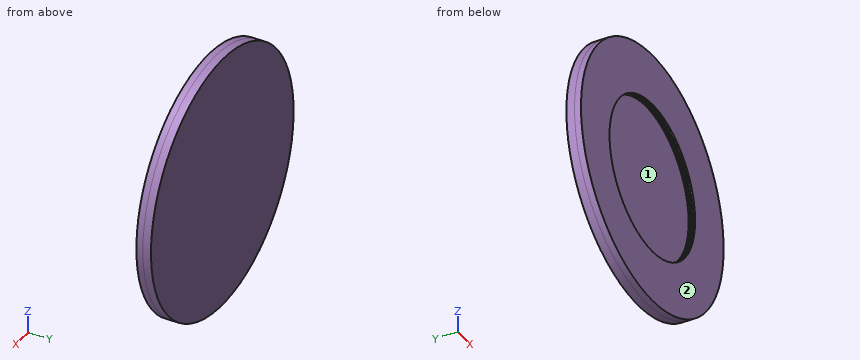
```python
from build123d import *

# Parameters (mm, degrees)
SKETCH1_R           = 15.875
BOSS_EXTRUDE1_DEPTH = 1
BOSS_EXTRUDE2_START = 0.8
SKETCH2_R           = 15.875
SKETCH2_R_2         = 9.525
BOSS_EXTRUDE2_DEPTH = 0.8
THREAD1_PITCH       = 0.25


with BuildPart() as part:
    # Sketch1 → Boss-Extrude1 (new body)
    with BuildSketch(Plane(origin=(0, 0, 0), x_dir=(1, 0, 0), z_dir=(0, 1, 0))):
        with Locations(Location((0, 0, 0), (0, 0, 270))):
            Circle(SKETCH1_R)
    extrude(amount=BOSS_EXTRUDE1_DEPTH)

    # Sketch2 → Boss-Extrude2 (add)
    with BuildSketch(Plane.XZ.offset(BOSS_EXTRUDE2_START)):
        with Locations(Location((0, 0, 0), (0, 0, 270))):
            Circle(SKETCH2_R)
        with Locations(Location((0, 0, 0), (0, 0, 270))):
            Circle(SKETCH2_R_2, mode=Mode.SUBTRACT)
    extrude(amount=-BOSS_EXTRUDE2_DEPTH)

    # Thread1: the profile of Thread Profile1 profile screwed along a right-hand helix of 4 turns, 6 arcs to a turn; built about Z, then put on its axis
    thread1_z = Axis((0, 0, 0), (0, 0, 1))
    thread1_corners = [(9.5247, 0, -0.000173205), (9.660316469, 0, 0.078125), (9.660316469, 0, 0.109375), (9.5247, 0, 0.187673204)]
    with BuildLine(mode=Mode.PRIVATE) as thread1_profile:
        Line(thread1_corners[0], thread1_corners[1])
        Line(thread1_corners[1], thread1_corners[2])
        Line(thread1_corners[2], thread1_corners[3])
        Line(thread1_corners[3], thread1_corners[0])
    thread1_cap = Face(thread1_profile.wire())
    thread1_turn_angles = [0, 30, 60, 90, 120, 150, 180, 210, 240, 270, 300, 330, 360]
    thread1_turn_weights = [1, 0.8660254037844387, 1, 0.8660254037844387, 1, 0.8660254037844387, 1, 0.8660254037844387, 1, 0.8660254037844387, 1, 0.8660254037844387, 1]
    thread1_turn_rails = [Edge.make_bspline([Vector(p[0], p[1], 0).rotate(thread1_z, thread1_turn_angles[k]) / thread1_turn_weights[k] + Vector(0, 0, p[2] + THREAD1_PITCH * thread1_turn_angles[k] / 360) for k in range(13)], [0, 0, 0, 1, 1, 2, 2, 3, 3, 4, 4, 5, 5, 6, 6, 6], 2, thread1_turn_weights) for p in thread1_corners]
    thread1_turn_sides = [Face.make_surface_from_curves(thread1_turn_rails[p[0]], thread1_turn_rails[p[1]]) for p in [(0, 1), (1, 2), (2, 3), (3, 0)]]
    thread1 = Plane(origin=(0, -0.8, 0), x_dir=(1, 0, 0), z_dir=(0, 1, 0)) * Solid(Shell([*[p.moved(Location((0, 0, THREAD1_PITCH * i))) for i in range(4) for p in thread1_turn_sides], thread1_cap, thread1_cap.rotate(thread1_z, 1440).moved(Location((0, 0, THREAD1_PITCH * 1440 / 360)))]))
    add(thread1, mode=Mode.SUBTRACT)


solid = part.part
```
Check sheet for the modelled part. Datum: model origin and axes. Units: mm. Face numbers are marked on the shaded views. Give positions to 0.01 mm unless a question says otherwise; leave off trailing zeros. Order: outer loops, then holes, each group sorted by start corner. A loop starts at its lowest first (then second) coordinate and runs counter-clockwise, first axis right, second up. Notation, with made-up numbers: (84.5, 65.5) -> (143.5, 65.5) arc R21 cw to (143.5, 94.5) -> close; hole circle Ø3 at (68, -24). An arc over 180 degrees is marked (long way). Use CSV: the item, a comma, the result in double quotes. Start each with the question number.
1) Mould release check, pull along X, two halves, no side actions. Record for the marked faces 1 and 2: released by +X, released by -X, zero draft, split by the parting line, or undercut.
2) Material ranges on line 1 (Y direction, x = -4.5, z = -2.5); line 2 (X direction, y = -0.25, z = 4); line 3 (Z direction, x = 0, y = -0.7) (3 decimals), recorded low to high. Write a range as from..to.
3) Go/stop test with flat-tipped pins: P1, Ø9.5, axis at x = -2.5, z = 1, coming from the -Y side; P2, Ø1, axis at x = 10.5, y = 0, coming from the +Z side. Record where each tip stops, or that it passes through.
4) Sectioned sample at A-A, the plane y = 0.7. Record the boundary of the cut face in (x, z) (3 decimals), plus the area to 3 significant figures.
5) Sectioned sample at D-D, the plane x = -12. Record the boundary of the cut face in (y, z), plus the area to 3 significant figures.
6) Sectioned sample at B-B, the plane z = 6.5. Give the number of separate pieces and of enclosed holes in the cut face, plus the area to 3 significant figures.
Recorded:
1,face 1,"undercut"
1,face 2,"zero draft"
2,line 1,"0..1"
2,line 2,"-15.36..-8.7, 8.77..15.36"
2,line 3,"-15.875..-9.59, 9.525..15.875"
3,P1,"y = 0"
3,P2,"z = 12.33"
4,outline,"circle Ø31.75 at (0, 0)"
4,area,"792 mm2"
5,outline,"(-0.8, -10.39) -> (1, -10.39) -> (1, 10.39) -> (-0.8, 10.39) -> close"
5,area,"37.4 mm2"
6,separate pieces,"1"
6,enclosed holes,"2"
6,area,"40.8 mm2"
